Check sheet for the drawn part. Datum: minimum x, y, z corner. Units: mm. A direction names the side the tool comes from. Coordinates: 2 decimals unless noted, no trailing zeros. Write each loop counter-clockwise with the first axis right and the second up, starting at its lowest first coordinate (ties: lowest second). Pieces come first, ordered by that corner, then holes. Notation, with made-up numbers: (65.5, -11) -> (69.5, -11) arc R6 cw to (69.5, -2) -> close; hole circle Ø7 at (15, 77). An arc over 180 degrees is marked (long way). Answer in a Markdown table with one row per item. Add a question column.
1. Cross-section at B-B on y = 16. Record the cut outline in (x, z) (3 decimals), and give its area (3 significant figures).
2. Cross-section at A-A on z = 4. Record the cut outline in (x, y) (3 decimals), and give its area (3 significant figures).
3. Cross-section at C-C on x = 6.75. Record the cut outline in (y, z), and give its area (3 significant figures).
4. Depth check by flat-ended pin: P1, Ø1.5, axis at x = 1.5, y = 14.5, coming from the +Z side; P2, Ø1, axis at x = 1, y = 13, coming from the +Z side; P3, Ø1, axis at y = 2.5, z = 6, coming from the +X side. Enter the tip coordinate at first touch or a pass-through.
5. Scan lines: L1, parallel to Y at x = 0.5, z = 5; L2, parallel to Y at x = 6.5, z = 3.5; L3, parallel to Z at x = 4, y = 3.5. Record each from-to range of solid material in increasing order. Write a range as from..to.
6. Mould release check, pull along Y, two halves, no side actions. Record for the marked faces 1, 2 and 3: pulls with the +Y half, pulls with the -Y half, needs draft (parallel to the pull), parting line crosses it, or undercut.
7. Set-up check for the marked faces 4, 5 and 6: record each of +Z, -Z, +X, -X, +Y, -Y from which the full face is reachable in a straight line by a thin tool's end or side.
8. Cross-section at D-D on y = 4.25. Record the cut outline in (x, z).
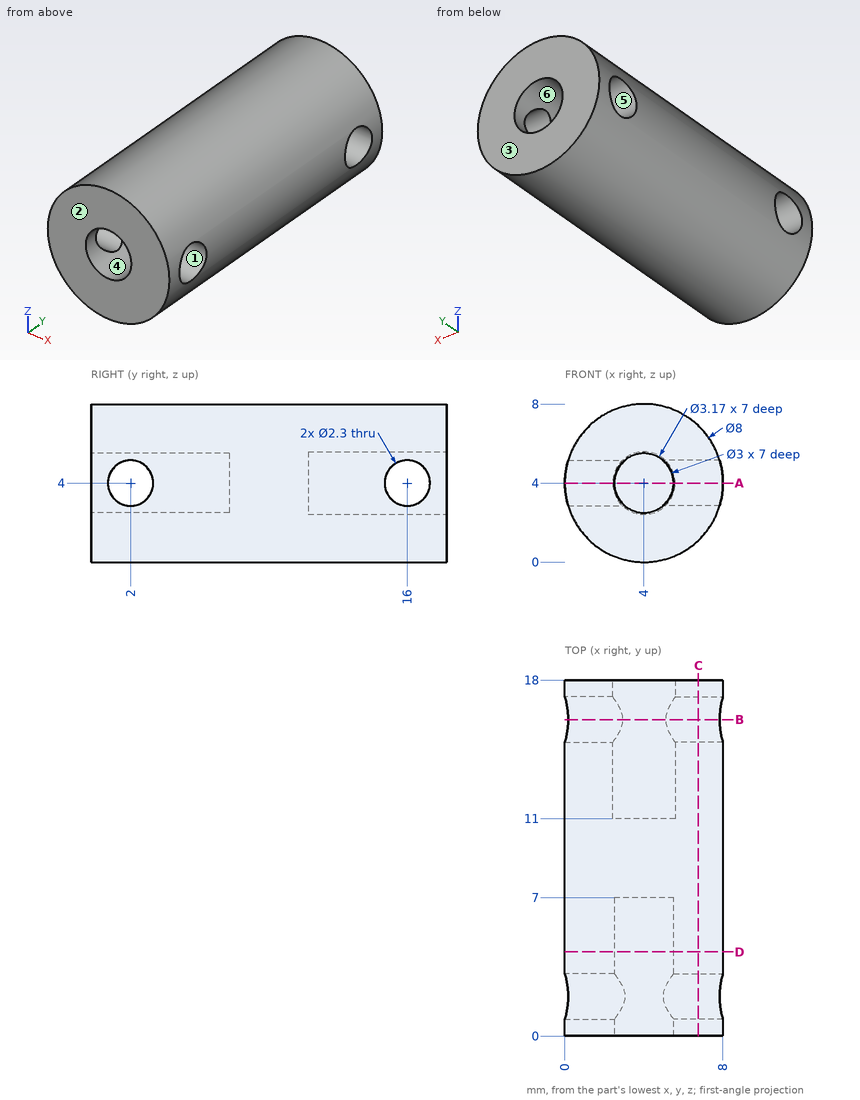
Results found:
| question | item | result |
|---|---|---|
| 1 | outline | (0.169, 2.85) arc R4 ccw to (7.831, 2.85) -> (5.091, 2.85) arc R1.585 cw to (2.909, 2.85) -> close; (0.169, 5.15) -> (2.909, 5.15) arc R1.585 cw to (5.091, 5.15) -> (7.831, 5.15) arc R4 ccw to start |
| 1 | area | 30.8 mm^2 |
| 2 | outline | (0, 0) -> (2.5, 0) -> (2.5, 0.85) -> (0, 0.85) -> close; (0, 3.15) -> (2.5, 3.15) -> (2.5, 7) -> (5.5, 7) -> (5.5, 3.15) -> (8, 3.15) -> (8, 14.85) -> (5.585, 14.85) -> (5.585, 11) -> (2.415, 11) -> (2.415, 14.85) -> (0, 14.85) -> close; (0, 17.15) -> (2.415, 17.15) -> (2.415, 18) -> (0, 18) -> close; (5.5, 0) -> (8, 0) -> (8, 0.85) -> (5.5, 0.85) -> close; (5.585, 17.15) -> (8, 17.15) -> (8, 18) -> (5.585, 18) -> close |
| 2 | area | 78.2 mm^2 |
| 3 | outline | (0, 1.1) -> (18, 1.1) -> (18, 6.9) -> (0, 6.9) -> close; hole circle Ø2.3 at (2, 4); hole circle Ø2.3 at (16, 4) |
| 3 | area | 96.3 mm^2 |
| 4 | P1 | stops at z = 7.6 |
| 4 | P2 | stops at z = 7.12 |
| 4 | P3 | stops at x = 7.71 |
| 5 | L1 | y = 0..1.43, 2.57..15.43, 16.57..18 |
| 5 | L2 | y = 0..0.96, 3.04..14.96, 17.04..18 |
| 5 | L3 | z = 0..2.5, 5.5..8 |
| 6 | face 1 | undercut |
| 6 | face 2 | pulls with the -Y half |
| 6 | face 3 | pulls with the +Y half |
| 7 | face 4 | -Y |
| 7 | face 5 | +X, -X |
| 7 | face 6 | +Y |
| 8 | outline | circle Ø8 at (4, 4); hole circle Ø3 at (4, 4) |
